Work out the finished part from the listing and answer in its coordinate system (mm). A direction names the side the tool comes from. Give positions to 0.01 mm unless a question says otherwise; leave off trailing zeros. Write each loop counter-clockwise with the first axis right and the second up, starting at its lowest first coordinate (ties: lowest second). Pieces come first, ordered by that corner, then holes.
1) A tool of negligible diameter and unlimited length cuts with its end or side. For faces 1 (the face through (35.45, 34.1, 0.86)), 2 (the face through (69, 17, 6)), from which of +Z, -Z, +X, -X, +Y, -Y can it reach the whole face along a straight path? Write none if from no direction.
2) Find section C-C (y = 21.5). Determine the outline of the cut face in (x, z).
3) Find section A-A (x = 6). Determine the outline of the cut face in (y, z).
4) Determine the mould class of faces 3 (the face through (35, 1, 6)), 4 (the face through (70, 17, 6)), 5 (the face through (34.55, 0.9, 0.86)) for opening direction X: pulls with the +X half, pulls with the -X half, needs draft (parallel to the pull), parting line crosses it, or undercut.
5) Given pin 1 Ø6 at (y, z) = (11.5, 8) entering from -X; pin 2 Ø10 at (x, y) = (44.5, 17) entering from +Z, each flat-ended and moving along its own axis, determine where each tip first touches the part or whether it passes through.
6) Find section B-B (z = 7.5). Determine the outline of the cut face in (x, y), plus the area to 3 significant figures.
7) Straight lines are drawn through the part: probe 1 along Y at (x, z) = (49.5, 8.5); probe 2 along X at (y, z) = (26.5, 5.75); probe 3 along Z at (x, y) = (55, 3). For each, find the intervals that lie inside material, in ascending order.
Autodesk Inventor part; units mm, degrees
ref_plane "YZ Plane" through (0, 0, 0) normal (1, 0, 0) x (0, 1, 0)
ref_plane "XZ Plane" through (0, 0, 0) normal (0, 1, 0) x (-1, 0, 0)
ref_plane "XY Plane" through (0, 0, 0) normal (0, 0, 1) x (1, 0, 0)
sketch "Esboço1" plane through (0, 0, 0) normal (0, 0, 1) x (1, 0, 0)
  line L0 (0, 0) -> (70, 0)
  line L1 (70, 0) -> (70, 35)
  line L2 (70, 35) -> (0, 35)
  line L3 (0, 35) -> (0, 0)
  dimension "d0" = 70
  dimension "d1" = 35
extrude "Extrusão1" add sketch "Esboço1" along normal blind 10
fillet "Arredondamento1" radius 3 4 edges at (70, 35, 5) (70, 0, 5) (0, 35, 5) (0, 0, 5)
fillet "Arredondamento2" radius 3 8 edges at (0.8787, 34.1213, 0) (0, 17.5, 0) (0.8787, 0.8787, 0) (35, 0, 0) (69.1213, 0.8787, 0) (70, 17.5, 0) (69.1213, 34.1213, 0) (35, 35, 0)
shell "Casca1" thickness 1 removed faces 1 at (45.6667, 11.6667, 10)
properties part number "Peça3-Rubia"
Results:
1. face 1: -Z, +X, -X, +Y
1. face 2: +Z
2. outline: (0, 3) arc R3 ccw to (3, 0) - (67, 0) arc R3 ccw to (70, 3) - (70, 10) - (69, 10) - (69, 3) arc R2 cw to (67, 1) - (3, 1) arc R2 cw to (1, 3) - (1, 10) - (0, 10) - close
3. outline: (0, 3) arc R3 ccw to (3, 0) - (32, 0) arc R3 ccw to (35, 3) - (35, 10) - (34, 10) - (34, 3) arc R2 cw to (32, 1) - (3, 1) arc R2 cw to (1, 3) - (1, 10) - (0, 10) - close
4. face 3: undercut
4. face 4: pulls with the +X half
4. face 5: needs draft
5. pin 1: stops at x = 0
5. pin 2: stops at z = 1
6. outline: (0, 3) arc R3 ccw to (3, 0) - (67, 0) arc R3 ccw to (70, 3) - (70, 32) arc R3 ccw to (67, 35) - (3, 35) arc R3 ccw to (0, 32) - close; hole (1, 3) arc R2 ccw to (3, 1) - (67, 1) arc R2 ccw to (69, 3) - (69, 32) arc R2 ccw to (67, 34) - (3, 34) arc R2 ccw to (1, 32) - close
6. area: 202 mm2
7. probe 1: y = 0 to 1, 34 to 35
7. probe 2: x = 0 to 1, 69 to 70
7. probe 3: z = 0 to 1
